```python
from build123d import *

# Parameters (mm, degrees)
F0_W           = 60
F0_H           = 30
F1_DEPTH       = 25
F2_R           = 5
F4_D           = 22
F4_CBORE_D     = 31.5
F4_CBORE_DEPTH = 20
F5_W           = 15
F5_H           = 10
F6_DEPTH       = 100.001
F7_W           = 15
F7_H           = 25
F8_DEPTH       = 60.001


with BuildPart() as f1:
    # F0 (on Front) → F1 (new body, symmetric)
    with BuildSketch(Plane.XZ):
        Polygon((-60, 60), (-100, 60), (-100, 0), (-60, 0), (-60, 30), align=None)
        with Locations((-30, 15)):
            Rectangle(F0_W, F0_H)
    extrude(amount=F1_DEPTH, both=True)

    # F2
    f2_edges = [f1.edges().sort_by_distance(p)[0] for p in [
        (-60, 0, 30),
        (-60, 0, 60),
        (0, 0, 30),
        (-100, 0, 60),
    ]]
    fillet(f2_edges, radius=F2_R)

    # F4 (through all)
    with Locations(Plane.XZ.offset(25)):
        with Locations((-78.1107470393, 36.7925874889)):
            CounterBoreHole(F4_D / 2, F4_CBORE_D / 2, F4_CBORE_DEPTH)

    # F5 (on face) → F6 (cut, through all)
    with BuildSketch(Plane.YZ):
        with Locations((0, 5)):
            Rectangle(F5_W, F5_H)
    extrude(amount=-F6_DEPTH, mode=Mode.SUBTRACT)

    # F7 (on face) → F8 (cut, through all)
    with BuildSketch(Plane.XY.offset(60)):
        Polygon((-80, 47.3070815206), (-123.8557249308, 47.3070815206), (-123.8557249308, 0), (-95, 0), (-95, 25), (-80, 25), align=None)
        with Locations((-87.5, 12.5)):
            Rectangle(F7_W, F7_H)
    extrude(amount=-F8_DEPTH, mode=Mode.SUBTRACT)


solid = f1.part
```
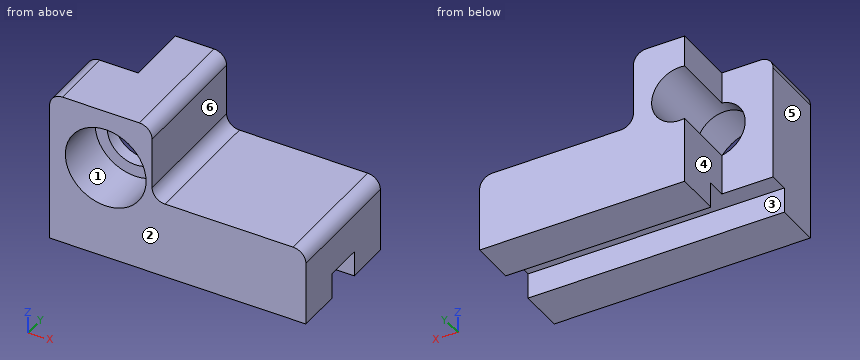
The listing builds one solid part. Answer for the finished solid, in the listing's coordinates (mm). Face numbers are marked on the shaded views. A direction names the side the tool comes from. Coordinates: 2 decimals unless noted, no trailing zeros. Write each loop counter-clockwise with the first axis right and the second up, starting at its lowest first coordinate (ties: lowest second). Pieces come first, ordered by that corner, then holes. Notation, with made-up numbers: M 79.5,87 L 96.5,87 A16 cw 96.5,102 Z; hole C 24.5,24 d6. An arc over 180 degrees is marked long. Use a Markdown table: item, result. Add a question column.
1. Section C-C (x = -20.5) is taken. Give the vertices of the cut face in (y, z).
2. Section B-B (y = 19) is taken. Give the vertices of the cut face in (x, z).
3. Section D-D (z = 50.5) is taken. Give the vertices of the cut face in (x, y), plus the area to 3 significant figures.
4. Straight lines are drawn through the part: line 1 along Y through (x, z) = (-46.5, 6); line 2 along Z through (x, y) = (-14.5, 10); line 3 along Z through (x, y) = (-29, -5). For each, find the intervals that lie inside material, in ascending order. Write a range as [from, to].
5. Section A-A (z = 7) is taken. Give the vertices of the cut face in (x, y).
6. For a pull along Y with two mould halves and no side action, classify the marked faces 1, 2 and 3 as +Y half, -Y half, draft (parallel to the pull), parting line (faces both ways), or undercut.
7. Which of the six approach directions +Z, -Z, +X, -X, +Y, -Y give full straight-line access (tool end or side, diameter ignored) to the marked faces 4, 5 and 6?
8. Given P1, Ø10, axis at y = 17, z = 56, coming from the -X side; P2, Ø15, axis at x = -34.5, y = -6.5, coming from the +Z side; P3, Ø9.5, axis at x = -71, z = 42.5, coming from the -Y side; P4, Ø20, axis at x = -78.11, z = 36.79, coming from the -Y side, each flat-ended and moving along its own axis, determine where each tip first touches the part or whether it passes through.
Data:
| question | item | result |
|---|---|---|
| 1 | outline | M -25,0 L -7.5,0 L -7.5,10 L 7.5,10 L 7.5,0 L 25,0 L 25,30 L -25,30 Z |
| 2 | outline | M -80,0 L 0,0 L 0,25 A5 ccw -5,30 L -55,30 A5 cw -60,35 L -60,55 A5 ccw -65,60 L -80,60 L -80,47.63 A11 cw long -80,25.96 Z |
| 3 | outline | M -100,-25 L -85.87,-25 L -85.87,-5 L -70.35,-5 L -70.35,-25 L -60,-25 L -60,25 L -80,25 L -80,0 L -100,0 Z |
| 3 | area | 1,190 mm2 |
| 4 | line 1 | y = [-25, -7.5], [7.5, 25] |
| 4 | line 2 | z = [0, 30] |
| 4 | line 3 | z = [10, 30] |
| 5 | outline | M -100,-25 L 0,-25 L 0,-7.5 L -100,-7.5 Z; M -80,7.5 L 0,7.5 L 0,25 L -80,25 Z |
| 6 | face 1 | draft |
| 6 | face 2 | -Y half |
| 6 | face 3 | undercut |
| 7 | face 4 | +Z, -Z, -X, +Y |
| 7 | face 5 | +Z, -Z, -X, +Y, -Y |
| 7 | face 6 | +Z, +X, +Y, -Y |
| 8 | P1 | stops at x = -80 |
| 8 | P2 | stops at z = 30 |
| 8 | P3 | stops at y = -5 |
| 8 | P4 | passes through |
